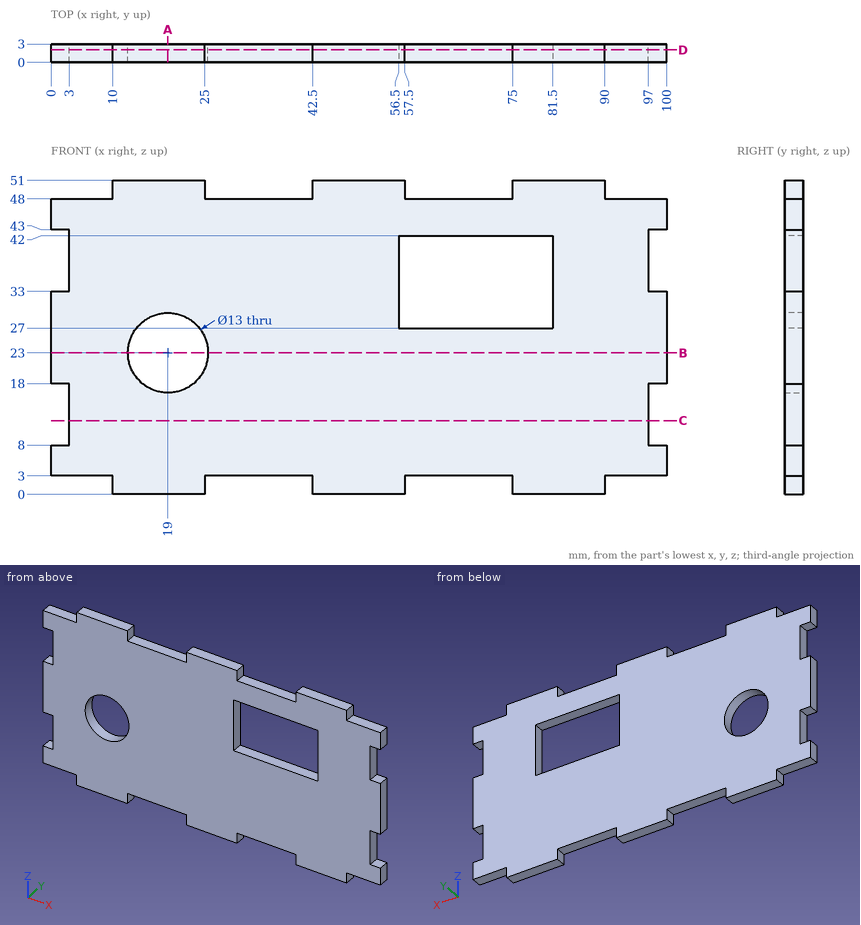
Part print with two shaded views. Sizes in mm from the minimum x, y, z corner. Round coordinates to 2 decimals unless told otherwise and drop trailing zeros. Write each loop counter-clockwise with the first axis right and the second up, starting at its lowest first coordinate (ties: lowest second). Pieces come first, ordered by that corner, then holes. Notation, with made-up numbers: (-23, 68.5) -> (-16, 68.5) arc R21 ccw to (-16, 101.5) -> close; hole circle Ø2 at (-34.75, 25). An arc over 180 degrees is marked (long way). Put each result on its own line as item: value.
Item 1: Slice it at B-B, the plane z = 23. Give the cut face in (x, y).
Here are the results:
outline: (0, 0) -> (12.5, 0) -> (12.5, 3) -> (0, 3) -> close; (25.5, 0) -> (100, 0) -> (100, 3) -> (25.5, 3) -> close
Item 2: Wall check: probe 1 along X at (y, z) = (0.55, 30); probe 2 along X at (y, z) = (2.2, 23); probe 3 along Z at (x, y) = (64, 1.1). Give the ranges that are in metal, low to high. Write a range as from..to.
Here are the results:
probe 1: x = 0..56.5, 81.5..100
probe 2: x = 0..12.5, 25.5..100
probe 3: z = 3..27, 42..48
Item 3: Flat gauge pins, fed straight in: P1, Ø0.9, axis at x = 99, y = 1.5, coming from the +Z side; P2, Ø1.5, axis at x = 3, y = 2, coming from the -Z side; P3, Ø0.9, axis at y = 2, z = 34, coming from the -X side. Where does each tip first touch, or does it go through?
Here are the results:
P1: stops at z = 48
P2: stops at z = 3
P3: stops at x = 3
Item 4: Slice it at C-C, the plane z = 12. Give the cut face in (x, y), plus the area to 3 significant figures.
Here are the results:
outline: (3, 0) -> (97, 0) -> (97, 3) -> (3, 3) -> close
area: 282 mm^2
Item 5: Slice it at D-D, the plane y = 2.05. Count the separate pieces of the cut face and the enclosed holes in it, plus the area to 3 significant figures.
Here are the results:
separate pieces: 1
enclosed holes: 2
area: 4,140 mm^2
Item 6: Slice it at A-A, the plane x = 19. Give the cut face in (y, z), plus the area to 3 significant figures.
Here are the results:
outline: (0, 0) -> (3, 0) -> (3, 16.5) -> (0, 16.5) -> close; (0, 29.5) -> (3, 29.5) -> (3, 51) -> (0, 51) -> close
area: 114 mm^2
